Autodesk Inventor part; units mm, degrees
ref_plane "Work Plane1" through (16.4368, 0, 0) normal (0, 0, 1) x (-1, 0, 0)
ref_plane "YZ Plane" through (0, 0, 0) normal (1, 0, 0) x (0, 1, 0)
ref_plane "XZ Plane" through (0, 0, 0) normal (0, 1, 0) x (-1, 0, 0)
sketch "Skizze1" plane through (0, 0, 0) normal (1, 0, 0) x (0, 1, 0)
  line L0 (2.8868, -5) -> (-2.8868, -5)
  line L1 (-2.8868, -5) -> (-5.7735, 0)
  line L2 (-5.7735, 0) -> (-2.8868, 5)
  line L3 (-2.8868, 5) -> (2.8868, 5)
  line L4 (2.8868, 5) -> (5.7735, 0)
  line L5 (5.7735, 0) -> (2.8868, -5)
  point P0 (0, 0)
  point P1 (0, 0)
  dimension "d0" = 11.547
extrude "Körper" add sketch "Skizze1" along normal blind 4
sketch "Skizze2" plane through (4, 0, 0) normal (1, 0, 0) x (0, 0, -1)
  circle A0 centre (0, 0) radius 4.45
  dimension "d7" = 8.9
extrude "Ring" add sketch "Skizze2" along normal blind 2
sketch "Skizze3" plane through (0, 0, 0) normal (0, 0, 1) x (1, 0, 0)
  line L0 (0, 2.8868) -> (0, 5.7735)
  line L1 (0, 5.7735) -> (4, 5.7735)
  line L2 (4, 2.8868) -> (4, 5.7735)
  line L3 (-0.8, 0) -> (4.8, 0)
  line L4 (0, 4.45) -> (0.7641, 5.7735)
  line L5 (3.2359, 5.7735) -> (4, 4.45)
  dimension "d3" = 30
  dimension "d4" = 30
  dimension "d5" = 8.9
  dimension "d6" = 8.9
revolve "Fase1" cut sketch "Skizze3" angle 360 about axis through (-10, 0, 0) along (1, 0, 0)
sketch "Skizze4" plane through (0, 0, 0) normal (-1, 0, 0) x (0, 0, 1)
  line L0 (0, -8.0829) -> (0, 8.0829)
  line L1 (-7, 0) -> (7, 0)
  point P0 (0, 0)
hole "Gewinde" at (0, 0, 0) direction (1, 0, 0) diameter 4.917 end through all
chamfer "Fase2" distance 0.5413 angle 30 1 edges at (0, 0, -2.4585) measured on face at (0, 3.7371, -0.4538)
chamfer "Fase3" distance 0.5413 angle 30 1 edges at (6, 0, -2.4585) measured on face at (6, -0.5511, -3.7193)
ref_plane "Work Plane1" through (16.4368, 0, 0) normal (0, 0, 1) x (-1, 0, 0)
equation "\"d0\" = 1.1547 * SW"
equation "\"d1\" = KOH1"
equation "\"d7\" = SD2"
equation "\"d8\" = KOH - KOH1"
equation "\"d3\" = ANG1"
equation "\"d4\" = ANG2"
equation "\"d5\" = SW0"
equation "\"d6\" = SW01"
equation "\"d10\" = -0.5 * GD1 + 0.5 * NND"
equation "\"d46\" = -0.5 * GD1 + 0.5 * NND"
equation "\"d12\" = -0.5 * GD1 + 0.5 * NND"
equation "\"d47\" = -0.5 * GD1 + 0.5 * NND"
equation "\"ANG1\" = 30deg"
equation "\"ANG2\" = 30deg"
equation "\"NND\" = 6"
equation "\"KOH1\" = 4"
equation "\"KOH\" = 6"
equation "\"SW0\" = 8.9"
equation "\"SW01\" = SW0"
equation "\"SD2\" = SW0"
equation "\"GUL\" = 0.541266 * PTC"
equation "\"THREADDIA\" = 6"
equation "\"TOA\" = 30deg"
equation "\"PTC\" = 1"
equation "\"GAL\" = 0.541266 * PTC"
equation "\"E0\" = 1.155 * SW"
properties part number "DIN 985 - M6" material "Stahl, weich"
Model file for the job. Use its own axes, mm. A direction names the side the tool comes from. Round coordinates to 2 decimals unless told otherwise and drop trailing zeros. Order: outer loops, then holes, each group sorted by start corner. A loop starts at its lowest first (then second) coordinate and runs counter-clockwise, first axis right, second up.
(1) Band-saw the part on C-C (x = 2.55). List the corners of the cut face in (y, z), then the cut area to 3 significant figures.
(2) Band-saw the part on D-D (x = 0.5). List the corners of the cut face in (y, z), then the cut area to 3 significant figures.
(3) Pull direction Y, two halves, no side cores. Call faces 3 (the face through (3.038, -0.738, 2.345)), 4 (the face through (1.976, -4.31, -2.535)), 5 (the face through (1.976, 4.31, 2.535)), 6 (the face through (6, -3, -1)): released by +Y, released by -Y, zero draft, split by the parting line, or undercut.
(4) Band-saw the part on B-B (x = 5.45). List the corners of the cut face in (y, z), then the cut area to 3 significant figures.
(5) Pin check, flat tips, straight feed: pin 1 (2 mm diameter, centred on x = 2, z = 3, fed in from -Y); pin 2 (5.5 mm diameter, centred on y = 0, z = 0, fed in from -X); pin 3 (1 mm diameter, centred on x = 3.5, z = -1, fed in from -Y). Stop position of each tip, or through.
(6) Band-saw the part on A-A (y = 0). List the corners of the cut face in (x, z).
(7) Drill centre lines: line 1 (Y direction, x = 4.45, z = 0); line 2 (Z direction, x = 3.4, y = 0); line 3 (Y direction, x = 4.15, z = -1.25). Where is each one in solid material? Low to high.
(8) 3-axis set-ups, long thin cutter, end or side, ignore diameter. For faces 1 (the face through (2, 0, -5)), 2 (the face through (4.986, 4.344, 0.965)): which of +Z, -Z, +X, -X, +Y, -Y reach the whole face in a straight line?
Verdict:
1. outline: (-5.77, 0) - (-2.89, -5) - (2.89, -5) - (5.77, 0) - (2.89, 5) - (-2.89, 5) - close; hole circle Ø4.92 at (0, 0)
1. area: 67.6 mm2
2. outline: (-5.23, -0.94) - (-3.43, -4.06) arc R5.32 ccw to (-1.81, -5) - (1.81, -5) arc R5.32 ccw to (3.43, -4.06) - (5.23, -0.94) arc R5.32 ccw to (5.23, 0.94) - (3.43, 4.06) arc R5.32 ccw to (1.81, 5) - (-1.81, 5) arc R5.32 ccw to (-3.43, 4.06) - (-5.23, 0.94) arc R5.32 ccw to start; hole circle Ø4.92 at (0, 0)
2. area: 65.2 mm2
3. face 3: undercut
3. face 4: released by -Y
3. face 5: released by +Y
3. face 6: zero draft
4. outline: circle Ø8.9 at (0, 0); hole circle Ø4.92 at (0, 0)
4. area: 43.2 mm2
5. pin 1: stops at y = -4.62
5. pin 2: stops at x = 0.14
5. pin 3: stops at y = -5.48
6. outline: (0, -4.45) - (0.32, -5) - (3.68, -5) - (4, -4.45) - (6, -4.45) - (6, -3) - (5.69, -2.46) - (0.31, -2.46) - (0, -3) - close; (0, 3) - (0.31, 2.46) - (5.69, 2.46) - (6, 3) - (6, 4.45) - (4, 4.45) - (3.68, 5) - (0.32, 5) - (0, 4.45) - close
7. line 1: y = -4.45 to -2.46, 2.46 to 4.45
7. line 2: z = -5 to -2.46, 2.46 to 5
7. line 3: y = -4.27 to -2.12, 2.12 to 4.27
8. face 1: -Z, +X, -X, +Y, -Y
8. face 2: +X
